Check sheet for the modelled part. Datum: model origin and axes. Units: mm. Round coordinates to 2 decimals unless told otherwise and drop trailing zeros. Order: outer loops, then holes, each group sorted by start corner. A loop starts at its lowest first (then second) coordinate and runs counter-clockwise, first axis right, second up. Notation, with made-up numbers: M 9.25,37.25 L 56.25,37.25 A20 cw 56.25,48.25 Z; hole C 7.5,16.25 d6. An arc over 180 degrees is marked long. One line per item, written item: value. Start each with the question number.
(1) Thickness scan on L1, parallel to Z at x = 0, y = -1.8; L2, parallel to X at y = -1.65, z = 25.4; L3, parallel to Z at x = -1, y = -2.15. Record the ranges inside material, lowest first.
(2) Cross-section at A-A, the plane z = 25.4. Enter the section's corners in (x, y), and give its area (3 significant figures).
(3) Release check for a two-part mould opening along X. For faces 1 (the face through (4, -4.63, 69)), 2 (the face through (19.05, -2, 71)), 3 (the face through (-0.675, -2.484, 71.994)), 4 (the face through (-19.05, -2, 71)) record: released by +X, released by -X, zero draft, split by the parting line, or undercut.
(4) Cross-section at B-B, the plane x = 0. Enter the section's corners in (y, z), and give its area (3 significant figures).
from build123d import *

# Parameters (mm, degrees)
BOSS_EXTRUDE1_DEPTH = 139.7
FILLET1_R           = 1.27
BOSS_EXTRUDE2_DEPTH = 25.4
FILLET2_R           = 1.27
FILLET3_R           = 1.27
FILLET4_R           = 1.27
SKETCH9_W           = 38.1
SKETCH9_H           = 139.7
BOSS_EXTRUDE3_DEPTH = 4.233333333
FILLET6_R           = 1.5875
FILLET7_R           = 0.396875
LPATTERN1_COUNT     = 2
LPATTERN1_PITCH     = 44.45
LPATTERN1_COL_COUNT = 2
LPATTERN1_COL_PITCH = 44.45
FILLET5_R           = 1.5875


with BuildPart() as part:
    # Sketch1 → Boss-Extrude1 (new body)
    with BuildSketch(Plane.XY):
        Polygon((-19.05, 0), (19.05, 0), (19.05, 12.7), (11.528846515, 12.7), (14.816666667, 4.7625), (-14.816666667, 4.7625), (-11.528846515, 12.7), (-19.05, 12.7), align=None)
    extrude(amount=BOSS_EXTRUDE1_DEPTH)

    # Fillet1
    fillet1_edges = [part.edges().sort_by_distance(p)[0] for p in [
        (-19.05, 12.7, 69.85),
        (-11.528846515, 12.7, 69.85),
        (-14.816666667, 4.7625, 69.85),
        (14.816666667, 4.7625, 69.85),
        (11.528846515, 12.7, 69.85),
        (19.05, 12.7, 69.85),
    ]]
    fillet(fillet1_edges, radius=FILLET1_R)

    # Fillet3
    fillet3_edges = [part.edges().sort_by_distance(p)[0] for p in [
        (19.05, 5.715, 0),
        (15.604767917, 12.7, 0),
        (15.604767917, 12.7, 139.7),
        (-19.05, 5.715, 0),
        (-15.604767917, 12.7, 0),
        (-13.172756591, 8.73125, 0),
        (0, 4.7625, 0),
        (13.172756591, 8.73125, 0),
        (-12.373569426, 12.135574196, 0),
        (-18.678025612, 12.328025612, 0),
        (12.373569426, 12.135574196, 0),
        (18.678025612, 12.328025612, 0),
        (13.172756591, 8.73125, 139.7),
        (0, 0, 139.7),
        (0, 4.7625, 139.7),
        (-13.172756591, 8.73125, 139.7),
        (-15.604767917, 12.7, 139.7),
        (-19.05, 5.715, 139.7),
        (-12.373569426, 12.135574196, 139.7),
        (-18.678025612, 12.328025612, 139.7),
        (12.373569426, 12.135574196, 139.7),
        (18.678025612, 12.328025612, 139.7),
        (13.971943756, 5.326925804, 0),
        (13.971943756, 5.326925804, 139.7),
        (-13.971943756, 5.326925804, 0),
        (-13.971943756, 5.326925804, 139.7),
        (19.05, 5.715, 139.7),
        (0, 0, 0),
    ]]
    fillet(fillet3_edges, radius=FILLET3_R)


with BuildPart() as body_2:
    # Sketch2 → Boss-Extrude2 (new body)
    with BuildSketch(Plane.XY.offset(139.7)):
        with BuildLine():
            Line((-11.904210726, 10.798189653), (11.904210726, 10.798189653))
            Line((11.904210726, 10.798189653), (13.737306252, 6.372705571))
            ThreePointArc((13.737306252, 6.372705571), (13.655153833, 5.538598063), (12.915977348, 5.1435))
            Line((12.915977348, 5.1435), (-12.915977348, 5.1435))
            ThreePointArc((-12.915977348, 5.1435), (-13.655153833, 5.538598063), (-13.737306252, 6.372705571))
            Line((-13.737306252, 6.372705571), (-11.904210726, 10.798189653))
        make_face()
    extrude(amount=BOSS_EXTRUDE2_DEPTH)

    # Fillet2
    fillet2_edges = [body_2.edges().sort_by_distance(p)[0] for p in [
        (-11.904210726, 10.798189653, 152.4),
        (11.904210726, 10.798189653, 152.4),
    ]]
    fillet(fillet2_edges, radius=FILLET2_R)

    # Fillet4
    fillet4_edges = [body_2.edges().sort_by_distance(p)[0] for p in [
        (-13.655153833, 5.538598063, 165.1),
        (0, 10.798189653, 139.7),
        (0, 10.798189653, 165.1),
        (0, 5.1435, 165.1),
        (-12.983128557, 8.193451592, 139.7),
        (-11.761198052, 10.584156061, 139.7),
        (11.761198052, 10.584156061, 139.7),
        (-12.983128557, 8.193451592, 165.1),
        (-11.761198052, 10.584156061, 165.1),
        (13.655153833, 5.538598063, 165.1),
        (11.761198052, 10.584156061, 165.1),
        (12.983128557, 8.193451592, 165.1),
        (13.655153833, 5.538598063, 139.7),
        (0, 5.1435, 139.7),
        (-13.655153833, 5.538598063, 139.7),
        (12.983128557, 8.193451592, 139.7),
    ]]
    fillet(fillet4_edges, radius=FILLET4_R)

    # Sketch4 → CSK for 1/4 Flat Head Machine Screw (100)1 (revolve, cut)
    with BuildSketch(Plane(origin=(0, 5.1435, 152.4), x_dir=(0, 0, -1), z_dir=(1, 0, 0))):
        Polygon((0, 0), (0, 7.5565), (3.3782, 7.5565), (3.3782, 2.568232241), (6.4389, 0), align=None)
    revolve(axis=Axis((0, -1.2065, 152.4), (0, 1, 0)), mode=Mode.SUBTRACT)


with BuildPart() as body_3:
    # Sketch9 → Boss-Extrude3 (new body)
    with BuildSketch(Plane(origin=(0, -0.396875, 0), x_dir=(-1, 0, 0), z_dir=(0, -1, 0))):
        with Locations((0, -69.85)):
            Rectangle(SKETCH9_W, SKETCH9_H)
    extrude(amount=BOSS_EXTRUDE3_DEPTH)

    # Fillet6
    fillet6_edges = [body_3.edges().sort_by_distance(p)[0] for p in [
        (19.05, -2.513541667, 0),
        (-19.05, -2.513541667, 0),
        (-19.05, -2.513541667, 139.7),
        (19.05, -2.513541667, 139.7),
    ]]
    fillet(fillet6_edges, radius=FILLET6_R)

    # Fillet7
    fillet7_edges = [body_3.edges().sort_by_distance(p)[0] for p in [
        (0, -0.396875, 139.7),
        (0, -4.630208333, 139.7),
        (19.05, -0.396875, 69.85),
        (0, -0.396875, 0),
        (-19.05, -0.396875, 69.85),
        (18.585032015, -0.396875, 0.464967985),
        (-18.585032015, -0.396875, 0.464967985),
        (-18.585032015, -0.396875, 139.235032015),
        (18.585032015, -0.396875, 139.235032015),
        (19.05, -4.630208333, 69.85),
        (-19.05, -4.630208333, 69.85),
        (0, -4.630208333, 0),
        (18.585032015, -4.630208333, 0.464967985),
        (-18.585032015, -4.630208333, 0.464967985),
        (-18.585032015, -4.630208333, 139.235032015),
        (18.585032015, -4.630208333, 139.235032015),
    ]]
    fillet(fillet7_edges, radius=FILLET7_R)


with BuildPart() as csk_for_8_flat_head_machine_screw_100_tool:
    # Sketch6 → CSK for #8 Flat Head Machine Screw (100)1 (revolve)
    with BuildSketch(Plane(origin=(0, 4.7625, 69.85), x_dir=(0, 0, 1), z_dir=(1, 0, 0))):
        Polygon((0, 0), (0, 9.392708333), (2.2479, 9.392708333), (2.2479, 1.651767624), (4.2164, 0), align=None)
    csk_for_8_flat_head_machine_screw_100 = revolve(axis=Axis((0, 11.1125, 69.85), (0, -1, 0)))


with BuildPart() as part_1:
    add(part.part)

    # CSK for #8 Flat Head Machine Screw (100)1: cut by csk_for_8_flat_head_machine_screw_100_tool
    add(csk_for_8_flat_head_machine_screw_100_tool.part, mode=Mode.SUBTRACT)


with BuildPart() as body_3_1:
    add(body_3.part)

    # CSK for #8 Flat Head Machine Screw (100)1: cut by csk_for_8_flat_head_machine_screw_100_tool
    add(csk_for_8_flat_head_machine_screw_100_tool.part, mode=Mode.SUBTRACT)


with BuildPart() as lpattern1_tool:
    # LPattern1: CSK for #8 Flat Head Machine Screw (100)1 ×2
    with Locations(*[(0, 0, i * LPATTERN1_PITCH) for i in range(1, LPATTERN1_COUNT)]):
        add(csk_for_8_flat_head_machine_screw_100)


with BuildPart() as part_2:
    add(part_1.part)

    # LPattern1: cut by lpattern1_tool
    add(lpattern1_tool.part, mode=Mode.SUBTRACT)


with BuildPart() as body_3_2:
    add(body_3_1.part)

    # LPattern1: cut by lpattern1_tool
    add(lpattern1_tool.part, mode=Mode.SUBTRACT)


with BuildPart() as lpattern1_col_tool:
    # LPattern1 col: CSK for #8 Flat Head Machine Screw (100)1 ×2
    with Locations(*[(0, 0, -i * LPATTERN1_COL_PITCH) for i in range(1, LPATTERN1_COL_COUNT)]):
        add(csk_for_8_flat_head_machine_screw_100)


with BuildPart() as part_3:
    add(part_2.part)

    # LPattern1 col: cut by lpattern1_col_tool
    add(lpattern1_col_tool.part, mode=Mode.SUBTRACT)

    # Fillet5
    fillet5_edges = [part_3.edges().sort_by_distance(p)[0] for p in [
        (0, 4.7625, 65.6336),
        (0, 4.7625, 21.1836),
        (0, 4.7625, 110.0836),
    ]]
    fillet(fillet5_edges, radius=FILLET5_R)


with BuildPart() as body_3_3:
    add(body_3_2.part)

    # LPattern1 col: cut by lpattern1_col_tool
    add(lpattern1_col_tool.part, mode=Mode.SUBTRACT)


solid = body_3_3.part
Values found:
1. L1: 0 to 23.15, 27.65 to 67.6, 72.1 to 112.05, 116.55 to 139.7
1. L2: -19.05 to -2.25, 2.25 to 19.05
1. L3: 0 to 23.39, 27.41 to 67.84, 71.86 to 112.29, 116.31 to 139.7
2. outline: M -19.05,-4.23 A0.4 ccw -18.65,-4.63 L -2.25,-4.63 L -2.25,-0.4 L -18.65,-0.4 A0.4 ccw -19.05,-0.79 Z; M 2.25,-4.63 L 18.65,-4.63 A0.4 ccw 19.05,-4.23 L 19.05,-0.79 A0.4 ccw 18.65,-0.4 L 2.25,-0.4 Z
2. area: 142 mm^2
3. face 1: zero draft
3. face 2: released by +X
3. face 3: undercut
3. face 4: released by -X
4. outline: M -4.63,0.4 A0.4 ccw -4.23,0 L -0.79,0 A0.4 ccw -0.4,0.4 L -0.4,23.15 L -4.63,23.15 Z; M -4.63,27.65 L -0.4,27.65 L -0.4,67.6 L -4.63,67.6 Z; M -4.63,72.1 L -0.4,72.1 L -0.4,112.05 L -4.63,112.05 Z; M -4.63,116.55 L -0.4,116.55 L -0.4,139.3 A0.4 ccw -0.79,139.7 L -4.23,139.7 A0.4 ccw -4.63,139.3 Z
4. area: 534 mm^2
